Here's how the part is built. I have some questions about the finished solid (model axes, mm). Coordinates: 2 decimals unless noted, no trailing zeros. Loops run counter-clockwise (first coordinate to the right, second up) from the corner with the lowest first, then second, coordinate; pieces in that order, holes last. Notation, with made-up numbers: M 54.25,13 L 60.25,13 A17 ccw 60.25,21 Z; hole C -19.75,-26.5 d7. An arc over 180 degrees is marked long. Use one line per item in the form item = value. Start each with the question number.
(1) Will these pins go through, and if not, where does the flat tip stop? P1, Ø0.6, axis at x = 16.5, y = -0.5, coming from the -Z side; P2, Ø0.6, axis at y = -0.5, z = -13, coming from the -X side; P3, Ø0.6, axis at x = 0, y = -0.5, coming from the +Z side.
(2) Thinking about a two-plate mould opening in X: for faces 1 (the flat face through (11, 0.762, -9)), 2 (the flat face through (11, 0, -9)), which applies, +X half, -X half, draft (parallel to the pull), parting line (faces both ways), or undercut?
(3) Imagine slicing it at C-C, the plane x = 14.75. Please give me the cut outline in (y, z).
(4) Imagine slicing it at B-B, the plane y = -0.25. Please give me the cut outline in (x, z).
(5) Imagine slicing it at A-A, the plane z = -11.75. Please give me the cut outline in (x, y), and give its area (3 significant figures).
(6) Please list where these lines run through material, in increasing order: L1, parallel to Z at x = 15.75, y = -0.05; L2, parallel to X at y = -0.4, z = -1; L3, parallel to Y at x = 22, z = -8.25.
```python
from build123d import *

# Parameters (mm, degrees)
SKETCH4_W           = 24.384
SKETCH4_H           = 19.558
BOSS_EXTRUDE1_DEPTH = 0.762
BOSS_EXTRUDE2_DEPTH = 0.762


with BuildPart() as part:
    # Sketch4 → Boss-Extrude1 (new body)
    with BuildSketch(Plane(origin=(0, 0, 0), x_dir=(1, 0, 0), z_dir=(0, 1, 0))):
        with Locations((11.43, 9.017)):
            Rectangle(SKETCH4_W, SKETCH4_H)
    extrude(amount=BOSS_EXTRUDE1_DEPTH)

    # Sketch6 → Boss-Extrude2 (add)
    with BuildSketch(Plane.XZ):
        Polygon((0, 0), (22.86, 0), (22.86, -18.034), (0, -18.034), (0, -12.192), (0.762, -12.192), (0.762, -17.272), (22.098, -17.272), (22.098, -0.762), (0.762, -0.762), (0.762, -5.842), (0, -5.842), align=None)
    extrude(amount=BOSS_EXTRUDE2_DEPTH)


solid = part.part
```
Answer:
q1.P1 = -18.03
q1.P2 = 0
q1.P3 = 0
q2.face_1 = draft
q2.face_2 = undercut
q3.outline = M -0.76,-18.03 L 0,-18.03 L 0,-18.8 L 0.76,-18.8 L 0.76,0.76 L 0,0.76 L 0,0 L -0.76,0 L -0.76,-0.76 L 0,-0.76 L 0,-17.27 L -0.76,-17.27 Z
q4.outline = M 0,-18.03 L 22.86,-18.03 L 22.86,0 L 0,0 L 0,-5.84 L 0.76,-5.84 L 0.76,-0.76 L 22.1,-0.76 L 22.1,-17.27 L 0.76,-17.27 L 0.76,-12.19 L 0,-12.19 Z
q5.outline = M -0.76,0 L 22.1,0 L 22.1,-0.76 L 22.86,-0.76 L 22.86,0 L 23.62,0 L 23.62,0.76 L -0.76,0.76 Z
q5.area = 19.2 mm²
q6.L1 = -18.03 to -17.27, -0.76 to 0
q6.L2 = 0 to 0.76, 22.1 to 22.86
q6.L3 = 0 to 0.76
